For this review, use the dimensioned drawing (mm, ordinates from the lowest corner) and the shaded views. Give positions to 0.01 mm unless a question says otherwise; leave off trailing zeros. Loops run counter-clockwise (first coordinate to the right, second up) from the corner with the lowest first, then second, coordinate; pieces in that order, holes last. Notation, with made-up numbers: (-23, -27) - (14, -27) arc R27 ccw to (14, -2) - close; hole circle Ø7 at (71.5, 66.5). An arc over 180 degrees is marked (long way). Put each result on its own line as item: value.
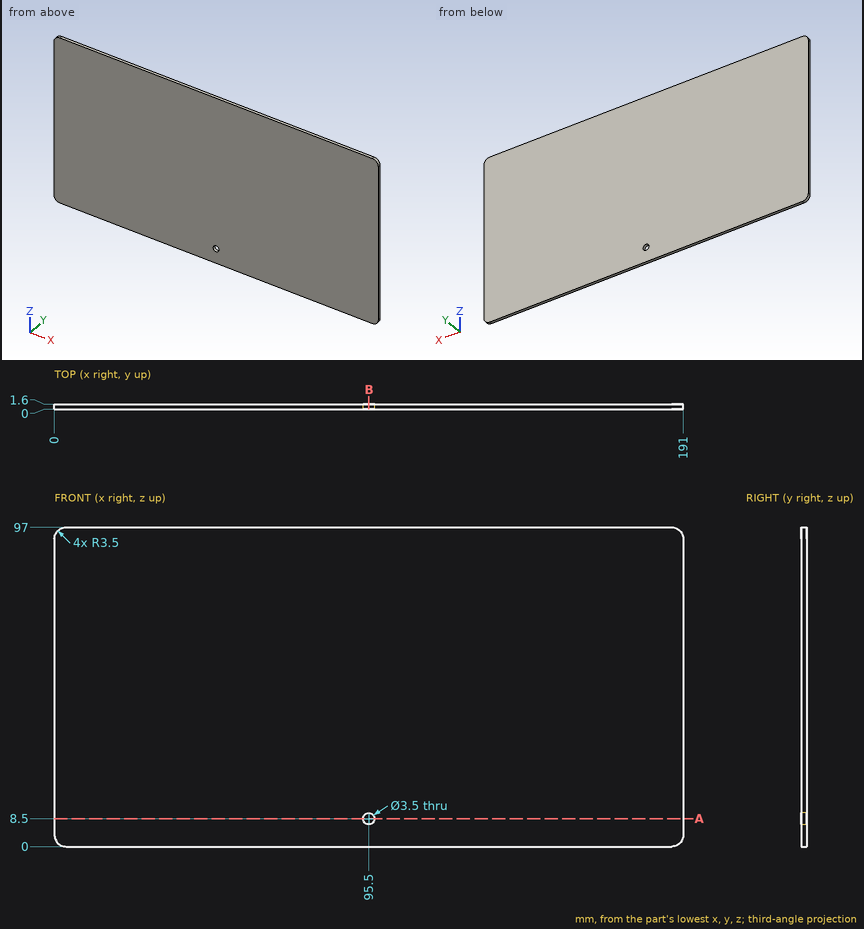
1) Take a section at B-B on x = 95.5. State the section outline as (y, z) points.
Geometry check:
outline: (0, 0) - (1.6, 0) - (1.6, 6.75) - (0, 6.75) - close; (0, 10.25) - (1.6, 10.25) - (1.6, 97) - (0, 97) - close
2) Take a section at A-A on z = 8.5. State the section outline as (x, y) points, and give its area (3 significant figures).
Geometry check:
outline: (0, 0) - (93.75, 0) - (93.75, 1.6) - (0, 1.6) - close; (97.25, 0) - (191, 0) - (191, 1.6) - (97.25, 1.6) - close
area: 300 mm²
3) Wall thickness on line 1 (X direction, y = 0.3, z = 8.5); line 2 (Z direction, x = 95.5, y = 1): over which ranges is each line inside the solid? List them lowest first.
Geometry check:
line 1: x = 0 to 93.75, 97.25 to 191
line 2: z = 0 to 6.75, 10.25 to 97
